Part model, mm, in its own coordinate system. Face numbers are marked on the shaded views. A direction names the side the tool comes from. Give positions to 0.01 mm unless a question says otherwise; leave off trailing zeros. Write each loop counter-clockwise with the first axis right and the second up, starting at its lowest first coordinate (ties: lowest second). Pieces come first, ordered by that corner, then holes. Notation, with made-up numbers: (-2, 86) - (24, 86) arc R19 ccw to (24, 116) - close; hole circle Ø3 at (-0.5, -10.5). An arc over 180 degrees is marked (long way). Answer in a Markdown table with one row per item. Add a question column.
1. Drop flat-ended pins along their axis: pin 1 Ø3 at (y, z) = (1.5, 18.5) entering from +X; pin 2 Ø5 at (y, z) = (3.5, 24) entering from +X; pin 3 Ø8 at (y, z) = (4.5, 26.5) entering from -X; pin 4 Ø2 at (y, z) = (-5, 22.5) entering from +X. Give the stop position or say it passes through.
2. Probe line 1 along X through (y, z) = (0.25, 20.5); line 2 along Z through (x, y) = (4, -1.5); line 3 along X through (y, z) = (-2.5, 3). List the from-to ranges inside material, lowest first.
3. Band-saw the part on A-A on y = 0. Write the cut outline in (x, z).
4. Band-saw the part on C-C on z = 10. Write the cut outline in (x, y), plus the area to 3 significant figures.
5. Which spindle directions (+Z, -Z, +X, -X, +Y, -Y) get a long thin tool onto all of the face, cutting with end or side? Do the marked faces 1 and 2. Say none if no direction does.
```python
from build123d import *

# Parameters (mm, degrees)
F0_R     = 4
F1_DEPTH = 6
F2_R     = 7
F2_R_2   = 4
F3_DEPTH = 25
F4_SIZE  = 2


with BuildPart() as f1:
    # F0 (on Top) → F1 (new body)
    with BuildSketch(Plane.XY):
        Circle(F0_R)
    extrude(amount=F1_DEPTH)

    # F2 (on face) → F3 (join)
    with BuildSketch(Plane.XY.offset(6)):
        Circle(F2_R)
        Circle(F2_R_2, mode=Mode.SUBTRACT)
        Circle(F2_R_2)
    extrude(amount=F3_DEPTH)

    # F4
    f4_edges = [f1.edges().sort_by_distance(p)[0] for p in [
        (-7, 0, 31),
    ]]
    chamfer(f4_edges, length=F4_SIZE)


solid = f1.part
```
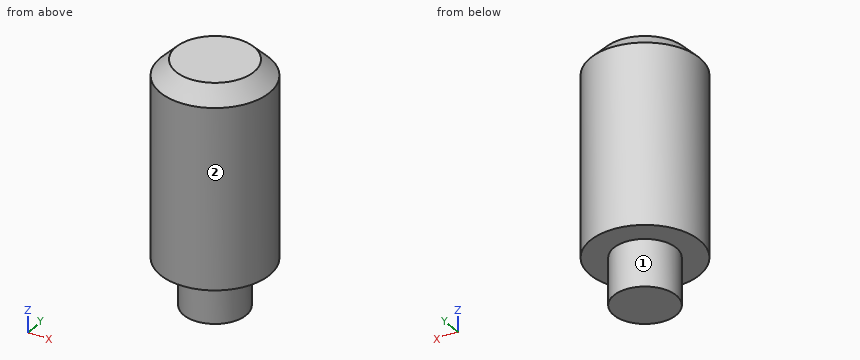
Values:
| question | item | result |
|---|---|---|
| 1 | pin 1 | stops at x = 7 |
| 1 | pin 2 | stops at x = 6.93 |
| 1 | pin 3 | stops at x = -6.98 |
| 1 | pin 4 | stops at x = 5.74 |
| 2 | line 1 | x = -7 to 7 |
| 2 | line 2 | z = 6 to 31 |
| 2 | line 3 | x = -3.12 to 3.12 |
| 3 | outline | (-7, 6) - (-4, 6) - (-4, 0) - (4, 0) - (4, 6) - (7, 6) - (7, 29) - (5, 31) - (-5, 31) - (-7, 29) - close |
| 4 | outline | circle Ø14 at (0, 0) |
| 4 | area | 154 mm² |
| 5 | face 1 | -Z |
| 5 | face 2 | +Z, -Z |
